The model under review builds one solid part; all positions refer to its coordinate system, in mm. A direction names the side the tool comes from. Coordinates: 2 decimals unless noted, no trailing zeros. Order: outer loops, then holes, each group sorted by start corner. A loop starts at its lowest first (then second) coordinate and runs counter-clockwise, first axis right, second up. Notation, with made-up numbers: (-11.75, 27.25) - (44.25, 27.25) arc R21 cw to (44.25, 64.25) - close; hole circle Ø10 at (-2, -14.75). An arc over 180 degrees is marked (long way). Answer in a Markdown table with one row per item.
```python
from build123d import *

# Parameters (mm, degrees)
SKETCH1_W           = 80
SKETCH1_H           = 36
BOSS_EXTRUDE1_DEPTH = 2
SKETCH2_R           = 1.5
CUT_EXTRUDE1_DEPTH  = 44.9089968
SKETCH3_W           = 71
SKETCH3_H           = 26
BOSS_EXTRUDE2_DEPTH = 8
CUT_EXTRUDE2_DEPTH  = 0.5
CUT_EXTRUDE3_DEPTH  = 0.1
BOSS_EXTRUDE3_DEPTH = 3
SKETCH10_R          = 0.5
CUT_EXTRUDE4_DEPTH  = 45.586993619


with BuildPart() as part:
    # Sketch1 → Boss-Extrude1 (new body)
    with BuildSketch(Plane(origin=(0, 0, 0), x_dir=(1, 0, 0), z_dir=(0, 1, 0))):
        Rectangle(SKETCH1_W, SKETCH1_H)
    extrude(amount=BOSS_EXTRUDE1_DEPTH)

    # Sketch2 → Cut-Extrude1 (cut, through all)
    with BuildSketch(Plane(origin=(0, 2, 0), x_dir=(1, 0, 0), z_dir=(0, 1, 0))):
        with Locations(Location((-37.5, 15.5, 0), (0, 0, 270))):
            Circle(SKETCH2_R)
        with Locations(Location((37.5, 15.5, 0), (0, 0, 90))):
            Circle(SKETCH2_R)
        with Locations(Location((-37.5, -15.5, 0), (0, 0, 90))):
            Circle(SKETCH2_R)
        with Locations(Location((37.5, -15.5, 0), (0, 0, 270))):
            Circle(SKETCH2_R)
    extrude(amount=-CUT_EXTRUDE1_DEPTH, mode=Mode.SUBTRACT)

    # Sketch3 → Boss-Extrude2 (add)
    with BuildSketch(Plane(origin=(0, 2, 0), x_dir=(1, 0, 0), z_dir=(0, 1, 0))):
        with Locations((0, -1)):
            Rectangle(SKETCH3_W, SKETCH3_H)
    extrude(amount=BOSS_EXTRUDE2_DEPTH)

    # Sketch5 → Cut-Extrude2 (cut)
    with BuildSketch(Plane(origin=(0, 10, 0), x_dir=(1, 0, 0), z_dir=(0, 1, 0))):
        with BuildLine():
            Line((-31.5, 7), (31.5, 7))
            ThreePointArc((31.5, 7), (32.207106781, 6.707106781), (32.5, 6))
            Line((32.5, 6), (32.5, -8))
            ThreePointArc((32.5, -8), (32.207106781, -8.707106781), (31.5, -9))
            Line((31.5, -9), (-31.5, -9))
            ThreePointArc((-31.5, -9), (-32.207106781, -8.707106781), (-32.5, -8))
            Line((-32.5, -8), (-32.5, 6))
            ThreePointArc((-32.5, 6), (-32.207106781, 6.707106781), (-31.5, 7))
        make_face()
    extrude(amount=-CUT_EXTRUDE2_DEPTH, mode=Mode.SUBTRACT)

    # Sketch6 → Cut-Extrude3 (cut)
    with BuildSketch(Plane(origin=(0, 10, 0), x_dir=(1, 0, 0), z_dir=(0, 1, 0))):
        with BuildLine():
            Line((33.01, 10), (-33.01, 10))
            ThreePointArc((-33.01, 10), (-33.356482323, 10.143517677), (-33.5, 10.49))
            Line((-33.5, 10.49), (-33.5, 10.51))
            ThreePointArc((-33.5, 10.51), (-33.356482323, 10.856482323), (-33.01, 11))
            Line((-33.01, 11), (33.01, 11))
            ThreePointArc((33.01, 11), (33.356482323, 10.856482323), (33.5, 10.51))
            Line((33.5, 10.51), (33.5, 10.49))
            ThreePointArc((33.5, 10.49), (33.356482323, 10.143517677), (33.01, 10))
        make_face()
        with BuildLine():
            Line((-33.5, -12.49), (-33.5, -12.51))
            ThreePointArc((-33.5, -12.51), (-33.356482323, -12.856482323), (-33.01, -13))
            Line((-33.01, -13), (33.01, -13))
            ThreePointArc((33.01, -13), (33.356482323, -12.856482323), (33.5, -12.51))
            Line((33.5, -12.51), (33.5, -12.49))
            ThreePointArc((33.5, -12.49), (33.356482323, -12.143517677), (33.01, -12))
            Line((33.01, -12), (-33.01, -12))
            ThreePointArc((-33.01, -12), (-33.356482323, -12.143517677), (-33.5, -12.49))
        make_face()
    extrude(amount=-CUT_EXTRUDE3_DEPTH, mode=Mode.SUBTRACT)

    # Sketch7 → Boss-Extrude3 (add)
    with BuildSketch(Plane(origin=(0, 2, 0), x_dir=(1, 0, 0), z_dir=(0, 1, 0))):
        Polygon((35.5, 8.5), (35.5, -10.5), (40, -4.249984615), (39.98, 2.249984615), align=None)
    extrude(amount=BOSS_EXTRUDE3_DEPTH)

    # Sketch10 → Cut-Extrude4 (cut, through all)
    with BuildSketch(Plane(origin=(0, 2, 0), x_dir=(1, 0, 0), z_dir=(0, 1, 0))):
        with Locations(Location((-32, 16, 0), (0, 0, 270))):
            Circle(SKETCH10_R)
        with Locations(Location((-29.5, 16, 0), (0, 0, 270))):
            Circle(SKETCH10_R)
        with Locations(Location((-27, 16, 0), (0, 0, 270))):
            Circle(SKETCH10_R)
        with Locations(Location((-24.5, 16, 0), (0, 0, 270))):
            Circle(SKETCH10_R)
        with Locations(Location((-22, 16, 0), (0, 0, 270))):
            Circle(SKETCH10_R)
        with Locations(Location((-19.5, 16, 0), (0, 0, 270))):
            Circle(SKETCH10_R)
        with Locations(Location((-17, 16, 0), (0, 0, 270))):
            Circle(SKETCH10_R)
        with Locations(Location((-14.5, 16, 0), (0, 0, 270))):
            Circle(SKETCH10_R)
        with Locations(Location((-12, 16, 0), (0, 0, 270))):
            Circle(SKETCH10_R)
        with Locations(Location((-9.5, 16, 0), (0, 0, 270))):
            Circle(SKETCH10_R)
        with Locations(Location((-7, 16, 0), (0, 0, 270))):
            Circle(SKETCH10_R)
        with Locations(Location((-4.5, 16, 0), (0, 0, 270))):
            Circle(SKETCH10_R)
        with Locations(Location((-2, 16, 0), (0, 0, 270))):
            Circle(SKETCH10_R)
        with Locations(Location((0.5, 16, 0), (0, 0, 270))):
            Circle(SKETCH10_R)
        with Locations(Location((3, 16, 0), (0, 0, 270))):
            Circle(SKETCH10_R)
        with Locations(Location((5.5, 16, 0), (0, 0, 270))):
            Circle(SKETCH10_R)
    extrude(amount=-CUT_EXTRUDE4_DEPTH, mode=Mode.SUBTRACT)


solid = part.part
```
Item 1: We need section C-C, the plane z = -4. Write out the cut boundary in (x, y), then the cut area to 3 significant figures.
Check values:
| item | result |
|---|---|
| outline | (-40, 0) - (40, 0) - (40, 2) - (38.73, 2) - (38.73, 5) - (35.5, 5) - (35.5, 10) - (32.5, 10) - (32.5, 9.5) - (-32.5, 9.5) - (-32.5, 10) - (-35.5, 10) - (-35.5, 2) - (-40, 2) - close |
| area | 705 mm^2 |
Item 2: Mouldability with a two-part tool opening along X and no side actions: class faces 1 (the face through (37.77, 3.48, -5.33)), 2 (the face through (-38.4, 1, -16.7)), 3 (the face through (-1, 0, 0)) as +X half, -X half, draft (parallel to the pull), parting line (faces both ways), or undercut.
Check values:
| item | result |
|---|---|
| face 1 | +X half |
| face 2 | undercut |
| face 3 | draft |
Item 3: Clearance check with flat-ended pins moving along their axes: pin 1 Ø2 at (x, y) = (-7.5, 8.5) entering from -Z; pin 2 Ø2.5 at (y, z) = (6, 1) entering from -X; pin 3 Ø5 at (x, y) = (3.5, 8.5) entering from +Z; pin 4 Ø2.5 at (x, z) = (-37.5, 15.5) entering from +Y. State where each tip first meets the part, or that it passes through.
Check values:
| item | result |
|---|---|
| pin 1 | z = -12 |
| pin 2 | x = -35.5 |
| pin 3 | z = 14 |
| pin 4 | through |
Item 4: We need section A-A, the plane x = 25. Write out the cut boundary in (y, z), then the cut area to 3 significant figures.
Check values:
| item | result |
|---|---|
| outline | (0, -18) - (2, -18) - (2, -12) - (10, -12) - (10, -11) - (9.9, -11) - (9.9, -10) - (10, -10) - (10, -7) - (9.5, -7) - (9.5, 9) - (10, 9) - (10, 12) - (9.9, 12) - (9.9, 13) - (10, 13) - (10, 14) - (2, 14) - (2, 18) - (0, 18) - close |
| area | 272 mm^2 |
Item 5: To check wall thickness, follow line 1 (X direction, y = 1.5, z = 15.5); line 2 (Y direction, x = -25.5, z = -5); line 3 (X direction, y = 7, z = -3). State the ranges of each line that lie inside material, in increasing order. Write a range as from..to.
Check values:
| item | result |
|---|---|
| line 1 | -40..-39, -36..36, 39..40 |
| line 2 | 0..9.5 |
| line 3 | -35.5..35.5 |
Item 6: We need section B-B, the plane y = 4. Write out the cut boundary in (x, z), then the cut area to 3 significant figures.
Check values:
| item | result |
|---|---|
| outline | (-35.5, -12) - (35.5, -12) - (35.5, -8.5) - (39.98, -2.25) - (40, 4.25) - (35.5, 10.5) - (35.5, 14) - (-35.5, 14) - close |
| area | 1,900 mm^2 |
Item 7: Tool access review of faces 4 (the face through (0, 6, 14)), 5 (the face through (37.72, 3.48, 7.42)), 6 (the face through (0, 6, -12)): name each direction out of +Z, -Z, +X, -X, +Y, -Y from which nothing blocks a thin tool from reaching the whole face with its end or side.
Check values:
| item | result |
|---|---|
| face 4 | +Z, +X, -X, +Y |
| face 5 | +Z, +X, +Y |
| face 6 | -Z, +X, -X, +Y |
